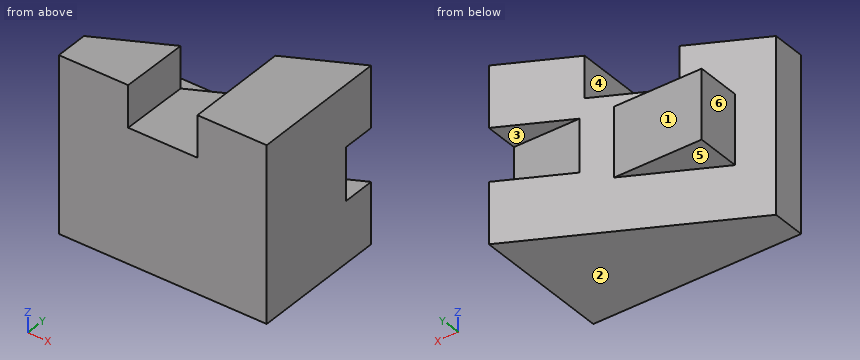
```python
from build123d import *

# Parameters (mm, degrees)
SKETCH2_W           = 75
SKETCH2_H           = 63
BOSS_EXTRUDE1_DEPTH = 50
CUT_EXTRUDE1_DEPTH  = 80
SKETCH6_W           = 19
SKETCH6_H           = 12
CUT_EXTRUDE2_DEPTH  = 80
CUT_EXTRUDE3_DEPTH  = 15
BOSS_EXTRUDE2_DEPTH = 12.5


with BuildPart() as part:
    # Sketch2 → Boss-Extrude1 (new body)
    with BuildSketch(Plane(origin=(0, 0, 0), x_dir=(1, 0, 0), z_dir=(0, 1, 0))):
        Rectangle(SKETCH2_W, SKETCH2_H)
    extrude(amount=BOSS_EXTRUDE1_DEPTH)

    # Sketch4 → Cut-Extrude1 (cut)
    with BuildSketch(Plane.XY.offset(31.5)):
        Polygon((-37.5, 12), (37.5, 50), (-37.5, 50), align=None)
    extrude(amount=-CUT_EXTRUDE1_DEPTH, mode=Mode.SUBTRACT)

    # Sketch6 → Cut-Extrude2 (cut)
    with BuildSketch(Plane(origin=(37.5, 0, 0), x_dir=(0, 0, -1), z_dir=(1, 0, 0))):
        with Locations((0, 44)):
            Rectangle(SKETCH6_W, SKETCH6_H)
    extrude(amount=-CUT_EXTRUDE2_DEPTH, mode=Mode.SUBTRACT)

    # Sketch8 → Cut-Extrude3 (cut)
    with BuildSketch(Plane.XY.offset(31.5)):
        Polygon((-12.253138509, 24.791743155), (-12.5, 0), (12.5, 0), (12.5, 37.333333333), align=None)
    extrude(amount=-CUT_EXTRUDE3_DEPTH, mode=Mode.SUBTRACT)

    # Sketch10 → Boss-Extrude2 (add, symmetric)
    with BuildSketch(Plane.XY):
        Polygon((4.783376681, 33.423577518), (-26.795570688, 17.423577518), (-26.795570688, 33.423577518), align=None)
    extrude(amount=BOSS_EXTRUDE2_DEPTH, both=True)


solid = part.part
```
Here's how the part is built. I have some questions about the finished solid (model axes, mm). Face numbers are marked on the shaded views. A direction names the side the tool comes from. Coordinates: 2 decimals unless noted, no trailing zeros. Order: outer loops, then holes, each group sorted by start corner. A loop starts at its lowest first (then second) coordinate and runs counter-clockwise, first axis right, second up. Notation, with made-up numbers: (58.25, -7.75) -> (112.25, -7.75) arc R19 cw to (112.25, 12.25) -> close; hole circle Ø7 at (13.5, 87). An arc over 180 degrees is marked (long way). Return JSON: item names as keys, results as strings.
1) If we section it at D-D on z = 4: List the corners of the cut face in (x, y) for me.
Conclusion:
{"outline": "(-37.5, 0) -> (37.5, 0) -> (37.5, 38) -> (13.82, 38) -> (4.78, 33.42) -> (-26.8, 33.42) -> (-26.8, 17.42) -> (-37.5, 12) -> close"}
2) If we section it at C-C on x = 27: List the corners of the cut face in (y, z) for me.
Conclusion:
{"outline": "(0, -31.5) -> (44.68, -31.5) -> (44.68, -9.5) -> (38, -9.5) -> (38, 9.5) -> (44.68, 9.5) -> (44.68, 31.5) -> (0, 31.5) -> close"}
3) On a 3-axis mill with a long thin cutter (end or side, diameter ignored), from which of +Z, -Z, +X, -X, +Y, -Y can I reach the whole of each face in a straight line? I mean the marked faces 4, 5 and 6. Say none if no direction works.
Conclusion:
{"face 4": "+Z, +Y, -Y", "face 5": "-Z, -X, +Y", "face 6": "+Z, -Z, -X, +Y"}
4) If I drill on probe 1 along Z at (x, y) = (28, 40.5); probe 2 along Z at (x, y) = (-16, 25.5); probe 3 along Z at (x, y) = (-5.5, 4.5), over which ranges is the centre line in solid material (lowest first)?
Conclusion:
{"probe 1": "z = -31.5 to -9.5, 9.5 to 31.5", "probe 2": "z = -12.5 to 12.5", "probe 3": "z = -31.5 to 16.5"}
5) If we section it at B-B on y = 39.5: List the corners of the cut face in (x, z) for me, plus the area to 3 significant figures.
Conclusion:
{"outline": "(16.78, -31.5) -> (37.5, -31.5) -> (37.5, -9.5) -> (16.78, -9.5) -> close; (16.78, 9.5) -> (37.5, 9.5) -> (37.5, 31.5) -> (16.78, 31.5) -> close", "area": "912 mm²"}
6) Thinking about a two-plate mould opening in Z: for the marked faces 1, 2 and 3, which applies, +Z half, -Z half, draft (parallel to the pull), parting line (faces both ways), or undercut?
Conclusion:
{"face 1": "draft", "face 2": "-Z half", "face 3": "undercut"}
7) If we section it at A-A on z = 27.5: List the corners of the cut face in (x, y) for me, plus the area to 3 significant figures.
Conclusion:
{"outline": "(-37.5, 0) -> (-12.5, 0) -> (-12.25, 24.79) -> (-37.5, 12) -> close; (12.5, 0) -> (37.5, 0) -> (37.5, 50) -> (12.5, 37.33) -> close", "area": "1,550 mm²"}
8) I'm going to push flat-ended pins straight in: P1, Ø8, axis at x = -29, y = 26, coming from the +Z side; P2, Ø20, axis at x = -14.5, z = -5, coming from the +Y side; P3, Ø13, axis at y = 21.5, z = 1, coming from the -X side; P4, Ø8, axis at x = 3, y = 40.5, coming from the +Z side. Where does each tip first touch, or does it pass through?
Conclusion:
{"P1": "stops at z = 12.5", "P2": "stops at y = 33.42", "P3": "stops at x = -31.58", "P4": "passes through"}
